from build123d import *

# Parameters (mm, degrees)
EXTRUDE1_DEPTH     = 110
CUT_EXTRUDE1_DEPTH = 81
EXTRUDE2_DEPTH     = 90
SKETCH4_W          = 71.56019469
SKETCH4_H          = 34.192707118
CUT_EXTRUDE2_DEPTH = 10


with BuildPart() as part:
    # Sketch1 → Extrude1 (new body)
    with BuildSketch(Plane.XY):
        Polygon((0, 0), (80, 0), (40, 28.008301528), align=None)
    extrude(amount=-EXTRUDE1_DEPTH)

    # Sketch2 → Cut-Extrude1 (cut, through all)
    with BuildSketch(Plane(origin=(0, 0, 0), x_dir=(0, 0, -1), z_dir=(1, 0, 0))):
        Polygon((0, 0), (19.611623863, 28.008301528), (0, 28.008301528), align=None)
    extrude(amount=CUT_EXTRUDE1_DEPTH, mode=Mode.SUBTRACT)

    # Sketch3 → Extrude2 (add)
    with BuildSketch(Plane(origin=(130, 0, 0), x_dir=(0, 0, -1), z_dir=(1, 0, 0))):
        Polygon((110, 0), (70, 0), (110, 40), align=None)
    extrude(amount=-EXTRUDE2_DEPTH)

    # Sketch4 → Cut-Extrude2 (cut)
    with BuildSketch(Plane(origin=(0, 0, 0), x_dir=(-0.819152044, -0.573576436, 0), z_dir=(-0.573576436, 0.819152044, 0))):
        with Locations((-35.780097345, -92.903646441)):
            Rectangle(SKETCH4_W, SKETCH4_H)
    extrude(amount=CUT_EXTRUDE2_DEPTH, mode=Mode.SUBTRACT)


solid = part.part
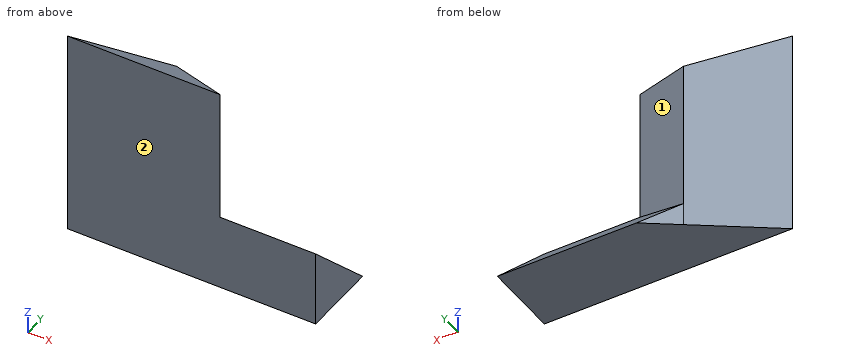
Model file for the job. Use its own axes, mm. Face numbers are marked on the shaded views. A direction names the side the tool comes from. Coordinates: 2 decimals unless noted, no trailing zeros. Write each loop counter-clockwise with the first axis right and the second up, starting at its lowest first coordinate (ties: lowest second). Pieces come first, ordered by that corner, then holes. Notation, with made-up numbers: (39.25, 61.5) -> (46.25, 61.5) arc R20 cw to (46.25, 84.5) -> close; hole circle Ø1 at (24.5, 89). An arc over 180 degrees is marked (long way). One line per item, written item: value. Start each with the question number.
1) Slice it at B-B on x = 100. Write the cut outline in (y, z), then the cut area to 3 significant figures.
2) Slice it at A-A on y = 24. Write the cut outline in (x, z), then the cut area to 3 significant figures.
3) Flat gauge pins, fed straight in: pin 1 Ø12 at (y, z) = (23.5, -91.5) entering from -X; pin 2 Ø1 at (y, z) = (21.5, -56.5) entering from -X; pin 3 Ø1 at (y, z) = (28, -60.5) entering from +X. Where does each tip first touch, or does it go through?
4) Slice it at D-D on y = 14.5. Write the cut outline in (x, z), then the cut area to 3 significant figures.
5) Probe probe 1 along X at (y, z) = (24.5, -83); probe 2 along Y at (x, z) = (92, -88); probe 3 along Z at (x, y) = (113.5, 17). List the from-to ranges inside material, lowest first.
6) Which spindle directions (+Z, -Z, +X, -X, +Y, -Y) get a long thin tool onto all of the face, cutting with end or side? Do the marked faces 1 and 2. Say none if no direction does.
7) Slice it at C-C on z = -86.5. Write the cut outline in (x, y).
Answers follow:
1. outline: (0, -110) -> (40, -110) -> (0, -70) -> close
1. area: 800 mm2
2. outline: (34.28, -110) -> (130, -110) -> (130, -94) -> (45.72, -94) -> (45.72, -16.8) -> (34.28, -16.8) -> close
2. area: 2,420 mm2
3. pin 1: x = 24.99
3. pin 2: x = 29.99
3. pin 3: x = 40.73
4. outline: (20.71, -110) -> (130, -110) -> (130, -84.5) -> (59.29, -84.5) -> (59.29, -10.15) -> (20.71, -10.15) -> close
4. area: 5,660 mm2
5. probe 1: 34.99 to 45.01
5. probe 2: 0 to 18
5. probe 3: -110 to -87
6. face 1: +Z, +X, +Y
6. face 2: +Z, -Z, +X, -X, -Y
7. outline: (0, 0) -> (130, 0) -> (130, 16.5) -> (56.44, 16.5) -> (40, 28.01) -> close
